Work out the finished part from the listing and answer in its coordinate system (mm). A direction names the side the tool comes from. Round coordinates to 2 decimals unless told otherwise and drop trailing zeros. Order: outer loops, then holes, each group sorted by start corner. A loop starts at its lowest first (then second) coordinate and runs counter-clockwise, first axis right, second up. Notation, with made-up numbers: (84, -26) -> (113, -26) arc R21 ccw to (113, 8) -> close; hole circle Ø6 at (82.5, 14). An arc over 180 degrees is marked (long way). Use one line per item in the form item = value.
```python
from build123d import *
from build123d.topology import SkipClean

# Parameters (mm, degrees)
BOSS_EXTRUDE1_DEPTH        = 10
BOSS_EXTRUDE1_DEPTH_BACK   = 10
BOSS_EXTRUDE1_2_DEPTH      = 10
BOSS_EXTRUDE1_2_DEPTH_BACK = 10
BOSS_EXTRUDE1_3_DEPTH      = 10
BOSS_EXTRUDE1_3_DEPTH_BACK = 10
BOSS_EXTRUDE1_4_DEPTH      = 10
BOSS_EXTRUDE1_4_DEPTH_BACK = 10
SKETCH2_R                  = 18
SKETCH2_R_2                = 14
BOSS_EXTRUDE2_DEPTH        = 4
BOSS_EXTRUDE3_START        = 4
SKETCH3_R                  = 18
SKETCH3_R_2                = 14
BOSS_EXTRUDE3_DEPTH        = 4
BOSS_EXTRUDE4_START        = 2.19
BOSS_EXTRUDE4_DEPTH        = 2.19
BOSS_EXTRUDE5_START        = 2
SKETCH5_R                  = 6
BOSS_EXTRUDE5_DEPTH        = 2
BOSS_EXTRUDE6_DEPTH        = 2.5
BOSS_EXTRUDE6_DEPTH_BACK   = 2.5


with BuildPart() as part:
    # Sketch1 → Boss-Extrude1 (new, two sides: drawn at the far end of the back side and taken through both)
    with BuildSketch(Plane.XY.offset(-BOSS_EXTRUDE1_DEPTH_BACK)):
        with BuildLine():
            Line((-2.491970197, -17.826667791), (-1.938199042, -13.86518606))
            ThreePointArc((-1.938199042, -13.86518606), (0, -14), (1.938199042, -13.86518606))
            Line((1.938199042, -13.86518606), (2.491970197, -17.826667791))
            ThreePointArc((2.491970197, -17.826667791), (0, -18), (-2.491970197, -17.826667791))
        make_face()
    extrude(amount=BOSS_EXTRUDE1_DEPTH + BOSS_EXTRUDE1_DEPTH_BACK)



with BuildPart() as body_2:
    # Sketch1 → Boss-Extrude1 2 (new, two sides: drawn at the far end of the back side and taken through both)
    with BuildSketch(Plane.XY.offset(-BOSS_EXTRUDE1_2_DEPTH_BACK)):
        with BuildLine():
            Line((-17.826667791, -2.491970197), (-13.86518606, -1.938199042))
            ThreePointArc((-13.86518606, -1.938199042), (-14, 0), (-13.86518606, 1.938199042))
            Line((-13.86518606, 1.938199042), (-17.826667791, 2.491970197))
            ThreePointArc((-17.826667791, 2.491970197), (-18, 0), (-17.826667791, -2.491970197))
        make_face()
    extrude(amount=BOSS_EXTRUDE1_2_DEPTH + BOSS_EXTRUDE1_2_DEPTH_BACK)


with BuildPart() as body_3:
    # Sketch1 → Boss-Extrude1 3 (new, two sides: drawn at the far end of the back side and taken through both)
    with BuildSketch(Plane.XY.offset(-BOSS_EXTRUDE1_3_DEPTH_BACK)):
        with BuildLine():
            Line((-2.491970197, 17.826667791), (-1.938199042, 13.86518606))
            ThreePointArc((-1.938199042, 13.86518606), (0, 14), (1.938199042, 13.86518606))
            Line((1.938199042, 13.86518606), (2.491970197, 17.826667791))
            ThreePointArc((2.491970197, 17.826667791), (0, 18), (-2.491970197, 17.826667791))
        make_face()
    extrude(amount=BOSS_EXTRUDE1_3_DEPTH + BOSS_EXTRUDE1_3_DEPTH_BACK)


with BuildPart() as body_4:
    # Sketch1 → Boss-Extrude1 4 (new, two sides: drawn at the far end of the back side and taken through both)
    with BuildSketch(Plane.XY.offset(-BOSS_EXTRUDE1_4_DEPTH_BACK)):
        with BuildLine():
            Line((17.826667791, -2.491970197), (13.86518606, -1.938199042))
            ThreePointArc((13.86518606, -1.938199042), (14, 0), (13.86518606, 1.938199042))
            Line((13.86518606, 1.938199042), (17.826667791, 2.491970197))
            ThreePointArc((17.826667791, 2.491970197), (18, 0), (17.826667791, -2.491970197))
        make_face()
    extrude(amount=BOSS_EXTRUDE1_4_DEPTH + BOSS_EXTRUDE1_4_DEPTH_BACK)


with BuildPart() as part_1:
    with SkipClean():  # the faces are left unmerged after this step: merging them gives an invalid solid
        add(part.part)

        add(body_2.part)  # Boss-Extrude2 merges body 2

        add(body_3.part)  # Boss-Extrude2 merges body 3

        add(body_4.part)  # Boss-Extrude2 merges body 4
        # Sketch2 → Boss-Extrude2 (add)
        with BuildSketch(Plane.XY.offset(10)):
            Circle(SKETCH2_R)
            Circle(SKETCH2_R_2, mode=Mode.SUBTRACT)
        extrude(amount=BOSS_EXTRUDE2_DEPTH)

    # Sketch3 → Boss-Extrude3 (add)
    with SkipClean():  # the faces are left unmerged after this step: merging them gives an invalid solid
        with BuildSketch(Plane(origin=(0, 0, -10), x_dir=(-1, 0, 0), z_dir=(0, 0, -1)).offset(BOSS_EXTRUDE3_START)):
            with Locations(Location((0, 0, 0), (0, 0, 180))):
                Circle(SKETCH3_R)
            with Locations(Location((0, 0, 0), (0, 0, 180))):
                Circle(SKETCH3_R_2, mode=Mode.SUBTRACT)
        extrude(amount=-BOSS_EXTRUDE3_DEPTH)

    # Sketch4 → Boss-Extrude4 (add)
    with SkipClean():  # the faces are left unmerged after this step: merging them gives an invalid solid
        with BuildSketch(Plane(origin=(0, 0, -14), x_dir=(-1, 0, 0), z_dir=(0, 0, -1)).offset(BOSS_EXTRUDE4_START)):
            with BuildLine():
                Line((10.843268656, -14.367446706), (8.433653399, -11.174680771))
                ThreePointArc((8.433653399, -11.174680771), (9.899494937, -9.899494937), (11.174680771, -8.433653399))
                Line((11.174680771, -8.433653399), (14.367446706, -10.843268656))
                ThreePointArc((14.367446706, -10.843268656), (12.727922061, -12.727922061), (10.843268656, -14.367446706))
            make_face()
            with BuildLine():
                Line((-10.843268656, -14.367446706), (-8.433653399, -11.174680771))
                ThreePointArc((-8.433653399, -11.174680771), (-9.899494937, -9.899494937), (-11.174680771, -8.433653399))
                Line((-11.174680771, -8.433653399), (-14.367446706, -10.843268656))
                ThreePointArc((-14.367446706, -10.843268656), (-12.727922061, -12.727922061), (-10.843268656, -14.367446706))
            make_face()
            with BuildLine():
                Line((14.367446706, 10.843268656), (11.174680771, 8.433653399))
                ThreePointArc((11.174680771, 8.433653399), (9.899494937, 9.899494937), (8.433653399, 11.174680771))
                Line((8.433653399, 11.174680771), (10.843268656, 14.367446706))
                ThreePointArc((10.843268656, 14.367446706), (12.727922061, 12.727922061), (14.367446706, 10.843268656))
            make_face()
            with BuildLine():
                Line((-8.433653399, 11.174680771), (-10.843268656, 14.367446706))
                ThreePointArc((-10.843268656, 14.367446706), (-12.727922061, 12.727922061), (-14.367446706, 10.843268656))
                Line((-14.367446706, 10.843268656), (-11.174680771, 8.433653399))
                ThreePointArc((-11.174680771, 8.433653399), (-9.899494937, 9.899494937), (-8.433653399, 11.174680771))
            make_face()
        extrude(amount=-BOSS_EXTRUDE4_DEPTH)

    # Sketch5 → Boss-Extrude5 (add)
    with SkipClean():  # the faces are left unmerged after this step: merging them gives an invalid solid
        with BuildSketch(Plane(origin=(0, 0, -16.19), x_dir=(-1, 0, 0), z_dir=(0, 0, -1)).offset(BOSS_EXTRUDE5_START)):
            with BuildLine():
                Line((-10.843268656, 14.367446706), (-4.819230514, 6.385531869))
                ThreePointArc((-4.819230514, 6.385531869), (0, 8), (4.819230514, 6.385531869))
                Line((4.819230514, 6.385531869), (10.843268656, 14.367446706))
                ThreePointArc((10.843268656, 14.367446706), (12.727922061, 12.727922061), (14.367446706, 10.843268656))
                Line((14.367446706, 10.843268656), (6.385531869, 4.819230514))
                ThreePointArc((6.385531869, 4.819230514), (7.008239781, 3.858053288), (7.487319643, 2.817808468))
                Line((7.487319643, 2.817808468), (9.3, 3.5))
                Line((9.3, 3.5), (12.2, 3.5))
                Line((12.2, 3.5), (12.7, 3))
                Line((12.7, 3), (12.7, 2.5))
                Line((12.7, 2.5), (12.2, 2))
                Line((12.2, 2), (10.8, 2))
                Line((10.8, 2), (10.8, -2))
                Line((10.8, -2), (12.2, -2))
                Line((12.2, -2), (12.7, -2.5))
                Line((12.7, -2.5), (12.7, -3))
                Line((12.7, -3), (12.2, -3.5))
                Line((12.2, -3.5), (9.3, -3.5))
                Line((9.3, -3.5), (7.487319643, -2.817808468))
                ThreePointArc((7.487319643, -2.817808468), (7.008239781, -3.858053288), (6.385531869, -4.819230514))
                Line((6.385531869, -4.819230514), (14.367446706, -10.843268656))
                ThreePointArc((14.367446706, -10.843268656), (12.727922061, -12.727922061), (10.843268656, -14.367446706))
                Line((10.843268656, -14.367446706), (4.819230514, -6.385531869))
                ThreePointArc((4.819230514, -6.385531869), (0, -8), (-4.819230514, -6.385531869))
                Line((-4.819230514, -6.385531869), (-10.843268656, -14.367446706))
                ThreePointArc((-10.843268656, -14.367446706), (-12.727922061, -12.727922061), (-14.367446706, -10.843268656))
                Line((-14.367446706, -10.843268656), (-6.385531869, -4.819230514))
                ThreePointArc((-6.385531869, -4.819230514), (-7.008239781, -3.858053288), (-7.487319643, -2.817808468))
                Line((-7.487319643, -2.817808468), (-9.3, -3.5))
                Line((-9.3, -3.5), (-12.2, -3.5))
                Line((-12.2, -3.5), (-12.7, -3))
                Line((-12.7, -3), (-12.7, -2.5))
                Line((-12.7, -2.5), (-12.2, -2))
                Line((-12.2, -2), (-10.8, -2))
                Line((-10.8, -2), (-10.8, 2))
                Line((-10.8, 2), (-12.2, 2))
                Line((-12.2, 2), (-12.7, 2.5))
                Line((-12.7, 2.5), (-12.7, 3))
                Line((-12.7, 3), (-12.2, 3.5))
                Line((-12.2, 3.5), (-9.3, 3.5))
                Line((-9.3, 3.5), (-7.487319643, 2.817808468))
                ThreePointArc((-7.487319643, 2.817808468), (-7.008239781, 3.858053288), (-6.385531869, 4.819230514))
                Line((-6.385531869, 4.819230514), (-14.367446706, 10.843268656))
                ThreePointArc((-14.367446706, 10.843268656), (-12.727922061, 12.727922061), (-10.843268656, 14.367446706))
            make_face()
            Circle(SKETCH5_R, mode=Mode.SUBTRACT)
        extrude(amount=-BOSS_EXTRUDE5_DEPTH)

    # Sketch6 → Boss-Extrude6 (add, two sides: drawn at the far end of the back side and taken through both)
    with SkipClean():  # the faces are left unmerged after this step: merging them gives an invalid solid
        with BuildSketch(Plane.XY.offset(-BOSS_EXTRUDE6_DEPTH_BACK)):
            with BuildLine():
                Line((-39, 2), (-15.874507866, 2))
                ThreePointArc((-15.874507866, 2), (-16, 0), (-15.874507866, -2))
                Line((-15.874507866, -2), (-39, -2))
                Line((-39, -2), (-39, 2))
            make_face()
            with BuildLine():
                Line((39, 2), (39, -2))
                Line((39, -2), (15.874507866, -2))
                ThreePointArc((15.874507866, -2), (16, 0), (15.874507866, 2))
                Line((15.874507866, 2), (39, 2))
            make_face()
            with BuildLine():
                Line((-2, 33), (2, 33))
                Line((2, 33), (2, 15.874507866))
                ThreePointArc((2, 15.874507866), (0, 16), (-2, 15.874507866))
                Line((-2, 15.874507866), (-2, 33))
            make_face()
            with BuildLine():
                Line((-2, -33), (2, -33))
                Line((2, -33), (2, -15.874507866))
                ThreePointArc((2, -15.874507866), (0, -16), (-2, -15.874507866))
                Line((-2, -15.874507866), (-2, -33))
            make_face()
        extrude(amount=BOSS_EXTRUDE6_DEPTH + BOSS_EXTRUDE6_DEPTH_BACK)


solid = part_1.part
```
Item 1: The part is cut by section C-C, the plane x = 0. Give the vertices of the cut face in (y, z), and give its area (3 significant figures).
Findings:
outline = (-33, -2.5) -> (-18, -2.5) -> (-18, -14) -> (-14, -14) -> (-14, 14) -> (-18, 14) -> (-18, 2.5) -> (-33, 2.5) -> close; (-8, -18.19) -> (-6, -18.19) -> (-6, -16.19) -> (-8, -16.19) -> close; (6, -18.19) -> (8, -18.19) -> (8, -16.19) -> (6, -16.19) -> close; (14, -14) -> (18, -14) -> (18, -2.5) -> (33, -2.5) -> (33, 2.5) -> (18, 2.5) -> (18, 14) -> (14, 14) -> close
area = 382 mm^2
Item 2: Flat-ended cylindrical pins translate along their axes: P1, Ø2.5, axis at y = 22, z = 0, coming from the -X side; P2, Ø19, axis at x = 0, y = 0, coming from the +Z side; P3, Ø5, axis at x = 29, y = 2, coming from the -Z side; P4, Ø8, axis at x = 25, y = -9, coming from the -Z side. Find the tip coordinate at first contact, or state that the pin passes through.
Findings:
P1 = -2
P2 = -16.19
P3 = -2.5
P4 = through
Item 3: For faces 1 (the flat face through (2.21, 15.82, -0.14)), 2 (the flat face through (29, 0, -2.5)), 3 (the flat face through (-8.406, -3.164, -17.204)), determine the directions among +Z, -Z, +X, -X, +Y, -Y from which every point of the face is accessible in a straight line to the end or side of a thin tool.
Findings:
face_1 = +X
face_2 = -Z, +X, +Y, -Y
face_3 = +Z, -Z
Item 4: Determine the mould class of faces 4 (the flat face through (-10.8, 0, -17)), 5 (the cylindrical face through (0, 8, -17)), 6 (the flat face through (0, -15, -14)) for opening direction Y: released by +Y, released by -Y, zero draft, split by the parting line, or undercut.
Findings:
face_4 = undercut
face_5 = released by +Y
face_6 = zero draft
Item 5: Consider line 1 along Y through (x, z) = (0, 10.85); line 2 along Y through (x, z) = (32.5, -1.5); line 3 along Z through (x, y) = (16, -2). Determine where each line is inside the solid, lowest interval first.
Findings:
line_1 = -18 to -14, 14 to 18
line_2 = -2 to 2
line_3 = -14 to 14
Item 6: The part is cut by section B-B, the plane z = -1. Give the number of separate pieces and of enclosed holes in the cut face, and give its area (3 significant figures).
Findings:
separate_pieces = 4
enclosed_holes = 0
area = 360 mm^2
Item 7: The part is cut by section D-D, the plane z = 12. Give the vertices of the cut face in (x, y), and give its area (3 significant figures).
Findings:
outline = circle Ø36 at (0, 0); hole circle Ø28 at (0, 0)
area = 402 mm^2
Item 8: The part is cut by section A-A, the plane y = 0. Give the vertices of the cut face in (x, z), and give its area (3 significant figures).
Findings:
outline = (-39, -2.5) -> (-18, -2.5) -> (-18, -14) -> (-14, -14) -> (-14, 14) -> (-18, 14) -> (-18, 2.5) -> (-39, 2.5) -> close; (-10.8, -18.19) -> (-6, -18.19) -> (-6, -16.19) -> (-10.8, -16.19) -> close; (6, -18.19) -> (10.8, -18.19) -> (10.8, -16.19) -> (6, -16.19) -> close; (14, -14) -> (18, -14) -> (18, -2.5) -> (39, -2.5) -> (39, 2.5) -> (18, 2.5) -> (18, 14) -> (14, 14) -> close
area = 453 mm^2
